Can you work these out from the model? Positions are in its coordinate system, mm. Coordinates: 2 decimals unless noted, no trailing zeros. Order: outer loops, then holes, each group sorted by start corner. A loop starts at its lowest first (then second) coordinate and runs counter-clockwise, first axis right, second up. Notation, with made-up numbers: M 61.5,73 L 119.5,73 A24 cw 119.5,96 Z; hole C 52,-26 d8. An arc over 180 degrees is marked long. Answer as CSV lines item,"result". Start each with the question number.
1. If we section it at A-A (x = 52): List the corners of the cut face in (y, z) for me.
2. If we section it at B-B (z = 135): Give the number of separate pieces and of enclosed holes in the cut face, plus the area to 3 significant figures.
3. Will these pins go through, and if not, where does the flat tip stop? pin 1 (1.5 mm diameter, centred on y = 33, z = 111, fed in from +X); pin 2 (3.5 mm diameter, centred on x = 35, z = 113.5, fed in from +Y); pin 3 (2.5 mm diameter, centred on y = 36.5, z = 62.5, fed in from -X).
4. I need wall thicknesses on line 1 along X through (y, z) = (37.5, 111); line 2 along X through (y, z) = (45.5, 215); line 3 along Y through (x, z) = (54, 97). Which ranges of each line are inside material? Lowest first, please. Write a range as from..to.
```python
from build123d import *

# Parameters (mm, degrees)
MODEL_R             = 2.100000001
BOSS_EXTRUDE1_DEPTH = 250


with BuildPart() as part:
    # Model → Boss-Extrude1 (new body)
    with BuildSketch(Plane.XY):
        with BuildLine():
            Line((28.771485975, 48.105572105), (30.646485975, 49.980572105))
            ThreePointArc((30.646485975, 49.980572105), (30.808697649, 50.08895848), (31.000039365, 50.127018713))
            Line((31.000039365, 50.127018713), (31.592932584, 50.127018713))
            Line((31.592932584, 50.127018713), (31.592932584, 47.752018713))
            Line((31.592932584, 47.752018713), (38.292932585, 47.752018713))
            ThreePointArc((38.292932585, 47.752018713), (38.505064619, 47.664150748), (38.592932584, 47.452018714))
            Line((38.592932584, 47.452018714), (38.592932584, 45.752018713))
            Line((38.592932584, 45.752018713), (35.592932585, 45.752018713))
            Line((35.592932585, 45.752018713), (35.592932585, 44.812678885))
            Line((35.592932585, 44.812678885), (38.653592756, 41.752018713))
            Line((38.653592756, 41.752018713), (41.292932583, 41.752018713))
            Line((41.292932583, 41.752018713), (41.592932584, 41.452018713))
            Line((41.592932584, 41.452018713), (41.892932586, 41.752018714))
            Line((41.892932586, 41.752018714), (44.532272412, 41.752018714))
            Line((44.532272412, 41.752018714), (47.592932584, 44.812678886))
            Line((47.592932584, 44.812678886), (47.592932584, 45.752018714))
            Line((47.592932584, 45.752018714), (44.592932584, 45.752018714))
            Line((44.592932584, 45.752018714), (44.592932584, 47.452018715))
            ThreePointArc((44.592932584, 47.452018715), (44.68080055, 47.664150749), (44.892932584, 47.752018715))
            Line((44.892932584, 47.752018715), (61.292932583, 47.752018715))
            Line((61.292932583, 47.752018715), (61.592932582, 47.452018715))
            Line((61.592932582, 47.452018715), (61.892932583, 47.752018716))
            Line((61.892932583, 47.752018716), (71.592932583, 47.752018716))
            Line((71.592932583, 47.752018716), (71.592932583, 50.127018711))
            Line((71.592932583, 50.127018711), (72.185825802, 50.127018711))
            ThreePointArc((72.185825802, 50.127018711), (72.377167518, 50.088958477), (72.539379192, 49.980572102))
            Line((72.539379192, 49.980572102), (74.414379192, 48.105572102))
            ThreePointArc((74.414379192, 48.105572102), (74.560825801, 47.752018712), (74.414379192, 47.398465322))
            Line((74.414379192, 47.398465322), (72.539379192, 45.523465322))
            ThreePointArc((72.539379192, 45.523465322), (72.377167518, 45.415078947), (72.185825802, 45.377018714))
            Line((72.185825802, 45.377018714), (72.092932582, 45.377018714))
            ThreePointArc((72.092932582, 45.377018714), (71.739379192, 45.230572103), (71.592932583, 44.877018713))
            Line((71.592932583, 44.877018713), (71.592932583, 41.052018712))
            ThreePointArc((71.592932583, 41.052018712), (71.505064617, 40.839886678), (71.292932581, 40.752018713))
            Line((71.292932581, 40.752018713), (69.592932583, 40.752018713))
            Line((69.592932583, 40.752018713), (69.592932583, 43.752018712))
            Line((69.592932583, 43.752018712), (68.653592755, 43.752018712))
            Line((68.653592755, 43.752018712), (65.592932583, 40.691358541))
            Line((65.592932583, 40.691358541), (65.592932583, 38.052018712))
            Line((65.592932583, 38.052018712), (65.292932584, 37.752018712))
            Line((65.292932584, 37.752018712), (65.592932583, 37.452018713))
            Line((65.592932583, 37.452018713), (65.592932583, 34.812678884))
            Line((65.592932583, 34.812678884), (68.653592755, 31.752018712))
            Line((68.653592755, 31.752018712), (69.592932583, 31.752018712))
            Line((69.592932583, 31.752018712), (69.592932583, 34.752018711))
            Line((69.592932583, 34.752018711), (71.292932581, 34.752018711))
            ThreePointArc((71.292932581, 34.752018711), (71.505064617, 34.664150747), (71.592932583, 34.452018712))
            Line((71.592932583, 34.452018712), (71.592932583, 28.75201871))
            ThreePointArc((71.592932583, 28.75201871), (71.300039364, 28.044911929), (70.592932582, 27.752018711))
            Line((70.592932582, 27.752018711), (64.892932582, 27.752018711))
            ThreePointArc((64.892932582, 27.752018711), (64.680800548, 27.839886676), (64.592932583, 28.05201871))
            Line((64.592932583, 28.05201871), (64.592932583, 29.752018711))
            Line((64.592932583, 29.752018711), (67.592932582, 29.752018711))
            Line((67.592932582, 29.752018711), (67.592932582, 30.69135854))
            Line((67.592932582, 30.69135854), (64.532272411, 33.752018711))
            Line((64.532272411, 33.752018711), (61.892932584, 33.752018711))
            Line((61.892932584, 33.752018711), (61.592932582, 34.052018713))
            Line((61.592932582, 34.052018713), (61.292932582, 33.752018712))
            Line((61.292932582, 33.752018712), (58.653592755, 33.752018712))
            Line((58.653592755, 33.752018712), (55.592932583, 30.691358541))
            Line((55.592932583, 30.691358541), (55.592932583, 29.752018713))
            Line((55.592932583, 29.752018713), (58.592932583, 29.752018713))
            Line((58.592932583, 29.752018713), (58.592932583, 28.052018712))
            ThreePointArc((58.592932583, 28.052018712), (58.505064617, 27.839886678), (58.292932583, 27.752018712))
            Line((58.292932583, 27.752018712), (44.892932584, 27.752018712))
            ThreePointArc((44.892932584, 27.752018712), (44.68080055, 27.839886678), (44.592932584, 28.052018712))
            Line((44.592932584, 28.052018712), (44.592932584, 29.752018713))
            Line((44.592932584, 29.752018713), (47.592932584, 29.752018713))
            Line((47.592932584, 29.752018713), (47.592932584, 30.691358541))
            Line((47.592932584, 30.691358541), (44.532272412, 33.752018712))
            Line((44.532272412, 33.752018712), (41.892932586, 33.752018712))
            Line((41.892932586, 33.752018712), (41.592932584, 34.052018714))
            Line((41.592932584, 34.052018714), (41.292932583, 33.752018714))
            Line((41.292932583, 33.752018714), (38.653592756, 33.752018714))
            Line((38.653592756, 33.752018714), (35.592932585, 30.691358542))
            Line((35.592932585, 30.691358542), (35.592932585, 29.752018714))
            Line((35.592932585, 29.752018714), (38.592932584, 29.752018714))
            Line((38.592932584, 29.752018714), (38.592932584, 28.052018713))
            ThreePointArc((38.592932584, 28.052018713), (38.505064619, 27.839886679), (38.292932585, 27.752018714))
            Line((38.292932585, 27.752018714), (32.592932585, 27.752018714))
            ThreePointArc((32.592932585, 27.752018714), (31.885825803, 28.044911931), (31.592932584, 28.752018713))
            Line((31.592932584, 28.752018713), (31.592932584, 34.452018715))
            ThreePointArc((31.592932584, 34.452018715), (31.68080055, 34.664150748), (31.892932583, 34.752018714))
            Line((31.892932583, 34.752018714), (33.592932584, 34.752018714))
            Line((33.592932584, 34.752018714), (33.592932584, 31.752018715))
            Line((33.592932584, 31.752018715), (34.532272412, 31.752018715))
            Line((34.532272412, 31.752018715), (37.592932584, 34.812678886))
            Line((37.592932584, 34.812678886), (37.592932584, 37.452018715))
            Line((37.592932584, 37.452018715), (37.892932583, 37.752018715))
            Line((37.892932583, 37.752018715), (37.592932584, 38.052018714))
            Line((37.592932584, 38.052018714), (37.592932584, 40.691358543))
            Line((37.592932584, 40.691358543), (34.532272412, 43.752018715))
            Line((34.532272412, 43.752018715), (33.592932584, 43.752018715))
            Line((33.592932584, 43.752018715), (33.592932584, 40.752018716))
            Line((33.592932584, 40.752018716), (31.892932586, 40.752018716))
            ThreePointArc((31.892932586, 40.752018716), (31.68080055, 40.83988668), (31.592932584, 41.052018715))
            Line((31.592932584, 41.052018715), (31.592932584, 44.877018715))
            ThreePointArc((31.592932584, 44.877018715), (31.446485975, 45.230572106), (31.092932585, 45.377018716))
            Line((31.092932585, 45.377018716), (31.000039365, 45.377018716))
            ThreePointArc((31.000039365, 45.377018716), (30.808697649, 45.41507895), (30.646485975, 45.523465324))
            Line((30.646485975, 45.523465324), (28.771485975, 47.398465325))
            ThreePointArc((28.771485975, 47.398465325), (28.625039366, 47.752018715), (28.771485975, 48.105572105))
        make_face()
        with Locations((61.592932582, 37.752018715)):
            Circle(MODEL_R, mode=Mode.SUBTRACT)
        with Locations((41.592932582, 37.752018715)):
            Circle(MODEL_R, mode=Mode.SUBTRACT)
        with BuildLine():
            Line((54.092932584, 29.752018715), (49.092932584, 29.752018715))
            Line((49.092932584, 29.752018715), (49.092932584, 31.312678886))
            Line((49.092932584, 31.312678886), (45.592932583, 34.812678886))
            Line((45.592932583, 34.812678886), (45.592932583, 40.691358543))
            Line((45.592932583, 40.691358543), (49.092932584, 44.191358544))
            Line((49.092932584, 44.191358544), (49.092932584, 45.752018714))
            Line((49.092932584, 45.752018714), (67.592932582, 45.752018714))
            Line((67.592932582, 45.752018714), (67.592932582, 44.812678887))
            Line((67.592932582, 44.812678887), (64.532272411, 41.752018716))
            Line((64.532272411, 41.752018716), (61.402932584, 41.752018716))
            ThreePointArc((61.402932584, 41.752018716), (58.708855747, 40.636095552), (57.592932584, 37.942018716))
            Line((57.592932584, 37.942018716), (57.592932584, 34.812678886))
            Line((57.592932584, 34.812678886), (54.092932584, 31.312678886))
            Line((54.092932584, 31.312678886), (54.092932584, 29.752018715))
        make_face(mode=Mode.SUBTRACT)
    extrude(amount=BOSS_EXTRUDE1_DEPTH)


solid = part.part
```
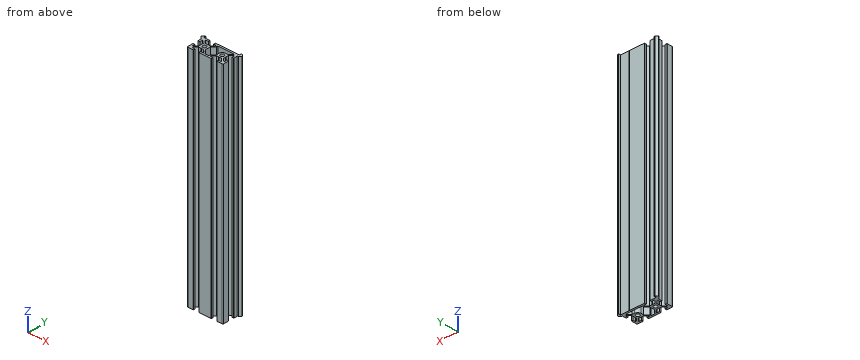
Solved:
1,outline,"M 27.75,0 L 29.75,0 L 29.75,250 L 27.75,250 Z; M 45.75,0 L 47.75,0 L 47.75,250 L 45.75,250 Z"
2,separate pieces,"1"
2,enclosed holes,"3"
2,area,"341 mm²"
3,pin 1,"x = 71.59"
3,pin 2,"y = 47.75"
3,pin 3,"x = 37.59"
4,line 1,"37.64..39.51, 43.68..45.59, 57.59..59.51, 63.68..65.54"
4,line 2,"30.67..35.59, 47.59..49.09, 67.59..72.51"
4,line 3,"27.75..29.75, 45.75..47.75"
